Model file for the job. Use its own axes, mm. Give positions to 0.01 mm unless a question says otherwise; leave off trailing zeros. Loops run counter-clockwise (first coordinate to the right, second up) from the corner with the lowest first, then second, coordinate; pieces in that order, holes last. Notation, with made-up numbers: (30.25, -17) - (38.25, -17) arc R12 cw to (38.25, -5) - close; hole circle Ø3 at (-19, 63). An arc over 180 degrees is marked (long way). Answer as CSV lines item,"result". Start each with the question number.
Item 1: Pull direction X, two halves, no side cores. Call faces 1 (the cylindrical face through (-9.644, 1.479, 6.825)), 2 (the flat face through (0, 0, 0)), 3 (the cylindrical face through (-21, 1, -28)): pulls with the +X half, pulls with the -X half, needs draft (parallel to the pull), parting line crosses it, or undercut.
Item 2: Pin check, flat tips, straight feed: pin 1 (1 mm diameter, centred on x = -17, y = 2, fed in from +Z); pin 2 (1.5 mm diameter, centred on x = -2, y = 2, fed in from -Z). Stop position of each tip, or through.
Item 3: Saw through at A-A on x = -7.5. Give the cut face in (y, z), plus the area to 3 significant figures.
Item 4: Saw through at B-B on y = 2.1. Give the cut face in (x, z).
Item 5: Saw through at D-D on z = 28. Give the cut face in (x, y), plus the area to 3 significant figures.
Item 6: Drill centre lines: L1, parallel to Z at x = 7.5, y = 0.8; L2, parallel to Z at x = 6.5, y = 0.35; L3, parallel to Z at x = 11.5, y = 2.5. Where is each one in solid material? Low to high. Write a range as from..to.
Item 7: Saw through at C-C on z = -7.5. Give the cut face in (x, y), plus the area to 3 significant figures.
from build123d import *

# Parameters (mm, degrees)
SKETCH1_R             = 35
BOSS_EXTRUDE1_DEPTH   = 3
F_8_CLEARANCE_HOLE1_D = 4.4958


with BuildPart() as part:
    # Sketch1 → Boss-Extrude1 (new body)
    with BuildSketch(Plane(origin=(0, 0, 0), x_dir=(1, 0, 0), z_dir=(0, 1, 0))):
        with Locations(Location((0, 0, 0), (0, 0, 270))):
            Circle(SKETCH1_R)
    extrude(amount=BOSS_EXTRUDE1_DEPTH)

    # #8 Clearance Hole1 (through all)
    with Locations(Plane(origin=(0, 3, 0), x_dir=(1, 0, 0), z_dir=(0, 1, 0))):
        with Locations((-7.5, 7.5), (7.5, 7.5), (-7.5, -7.5), (7.5, -7.5)):
            Hole(F_8_CLEARANCE_HOLE1_D / 2)


solid = part.part
Responses:
1,face 1,"undercut"
1,face 2,"needs draft"
1,face 3,"parting line crosses it"
2,pin 1,"z = 30.87"
2,pin 2,"z = -34.98"
3,outline,"(0, -34.19) - (3, -34.19) - (3, -9.75) - (0, -9.75) - close; (0, -5.25) - (3, -5.25) - (3, 5.25) - (0, 5.25) - close; (0, 9.75) - (3, 9.75) - (3, 34.19) - (0, 34.19) - close"
3,area,"178 mm2"
4,outline,"circle Ø70 at (0, 0); hole circle Ø4.5 at (-7.5, -7.5); hole circle Ø4.5 at (-7.5, 7.5); hole circle Ø4.5 at (7.5, -7.5); hole circle Ø4.5 at (7.5, 7.5)"
5,outline,"(-21, 0) - (21, 0) - (21, 3) - (-21, 3) - close"
5,area,"126 mm2"
6,L1,"-34.19..-9.75, -5.25..5.25, 9.75..34.19"
6,L2,"-34.39..-9.51, -5.49..5.49, 9.51..34.39"
6,L3,"-33.06..33.06"
7,outline,"(-34.19, 0) - (-9.75, 0) - (-9.75, 3) - (-34.19, 3) - close; (-5.25, 0) - (5.25, 0) - (5.25, 3) - (-5.25, 3) - close; (9.75, 0) - (34.19, 0) - (34.19, 3) - (9.75, 3) - close"
7,area,"178 mm2"
